Verification items for the finished model (mm, model axes). Coordinates: 2 decimals unless noted, no trailing zeros. Loops run counter-clockwise (first coordinate to the right, second up) from the corner with the lowest first, then second, coordinate; pieces in that order, holes last. Notation, with made-up numbers: (-14, -20.5) - (1, -20.5) arc R26 ccw to (1, 2.5) - close; hole circle Ø5 at (79.5, 60.25). An arc over 180 degrees is marked (long way). Answer as CSV lines item,"result". Start each with the question number.
1. Release check for a two-part mould opening along Z. For faces 1 (the cylindrical face through (-0.635, 0.525, -4.834)), 2 (the flat face through (0, -37.5, 0)), 3 (the flat face through (0, 36, -3.15)) record: pulls with the +Z half, pulls with the -Z half, needs draft (parallel to the pull), parting line crosses it, or undercut.
2. Material ranges on line 1 (Y direction, x = 2, z = 2); line 2 (X direction, y = 15.5, z = -0.25), recorded low to high. Write a range as [from, to].
3. Cross-section at A-A (z = 0). Enter the section's corners in (x, y) (3 decimals), plus the area to 4 significant figures.
4. Gauge pin test, flat ends, axial feed: P1, Ø2, axis at x = -3, y = -13.5, coming from the -Z side; P2, Ø3, axis at x = 1, z = 0.5, coming from the +Y side; P3, Ø1.2, axis at y = 36, z = -1.5, coming from the +X side. Record the tip position at first contact, or that the pin passes through.
5. Cross-section at D-D (x = -4). Enter the section's corners in (y, z).
6. Cross-section at C-C (y = 9.5). Enter the section's corners in (x, z) (3 decimals).
7. Cross-section at B-B (x = 0). Enter the section's corners in (y, z) (3 decimals).
```python
from build123d import *

# Parameters (mm, degrees)
SKETCH1_R           = 4.875
BOSS_EXTRUDE1_DEPTH = 37.5
SKETCH2_W           = 6.3
SKETCH2_H           = 6.3
BOSS_EXTRUDE2_DEPTH = 2.5
SKETCH3_W           = 6.3
SKETCH3_H           = 6.3
CUT_EXTRUDE1_DEPTH  = 5


with BuildPart() as part:
    # Sketch1 → Boss-Extrude1 (new body, symmetric)
    with BuildSketch(Plane(origin=(0, 0, 0), x_dir=(1, 0, 0), z_dir=(0, 1, 0))):
        Circle(SKETCH1_R)
    extrude(amount=BOSS_EXTRUDE1_DEPTH, both=True)

    # Sketch2 → Boss-Extrude2 (add)
    with BuildSketch(Plane(origin=(0, 37.5, 0), x_dir=(1, 0, 0), z_dir=(0, 1, 0))):
        Rectangle(SKETCH2_W, SKETCH2_H)
    extrude(amount=BOSS_EXTRUDE2_DEPTH)

    # Sketch3 → Cut-Extrude1 (cut)
    with BuildSketch(Plane(origin=(0, 40, 0), x_dir=(1, 0, 0), z_dir=(0, 1, 0))):
        Rectangle(SKETCH3_W, SKETCH3_H)
    extrude(amount=-CUT_EXTRUDE1_DEPTH, mode=Mode.SUBTRACT)


solid = part.part
```
Values follow:
1,face 1,"parting line crosses it"
1,face 2,"needs draft"
1,face 3,"undercut"
2,line 1,"y = [-37.5, 35]"
2,line 2,"x = [-4.87, 4.87]"
3,outline,"(-4.875, -37.5) - (4.875, -37.5) - (4.875, 37.5) - (3.15, 37.5) - (3.15, 35) - (-3.15, 35) - (-3.15, 37.5) - (-4.875, 37.5) - close"
3,area,"715.5 mm²"
4,P1,"stops at z = -4.45"
4,P2,"stops at y = 35"
4,P3,"stops at x = 4.79"
5,outline,"(-37.5, -2.79) - (37.5, -2.79) - (37.5, 2.79) - (-37.5, 2.79) - close"
6,outline,"circle Ø9.75 at (0, 0)"
7,outline,"(-37.5, -4.875) - (37.5, -4.875) - (37.5, -3.15) - (35, -3.15) - (35, 3.15) - (37.5, 3.15) - (37.5, 4.875) - (-37.5, 4.875) - close"
